Design review of the part built by this model. Coordinates are the model's own, in mm. A direction names the side the tool comes from. Coordinates: 2 decimals unless noted, no trailing zeros. Write each loop counter-clockwise with the first axis right and the second up, starting at its lowest first coordinate (ties: lowest second). Pieces come first, ordered by that corner, then holes. Notation, with made-up numbers: M 89,83 L 132,83 A26 cw 132,119 Z; hole C 77,-22 d10. An arc over 180 degrees is marked long. Write item = value, one per line.
```python
from build123d import *

# Parameters (mm, degrees)
SKETCH_1_W               = 400
SKETCH_1_H               = 150
EXTRUDE_1_DEPTH          = 300
SKETCH_2_R               = 30
EXTRUDE_2_DEPTH          = 20
SKETCH_8_W               = 200
SKETCH_8_H               = 15
EXTRUDE_6_DEPTH          = 80
SKETCH_9_R               = 20
EXTRUDE_7_DEPTH          = 20
MIRROR_4_COPY_1_SKETCH_R = 20
MIRROR_4_COPY_1_DEPTH    = 20
SKETCH_10_R              = 2
CUT_EXTRUDE_1_DEPTH      = 10
EXTRUDE_START            = 20
SKETCH_6_R               = 30
EXTRUDE_8_DEPTH          = 20


with BuildPart() as part:
    # 草图1 → 凸台-拉伸1 (new body)
    with BuildSketch(Plane.XY):
        Rectangle(SKETCH_1_W, SKETCH_1_H)
    extrude(amount=-EXTRUDE_1_DEPTH)

    # 草图2 → 凸台-拉伸2 (add)
    with BuildSketch(Plane(origin=(200, 0, 0), x_dir=(0, 0, -1), z_dir=(1, 0, 0))):
        with Locations(Location((150, 0, 0), (0, 0, 90))):
            Circle(SKETCH_2_R)
    extrude(amount=EXTRUDE_2_DEPTH)

    # 草图8 → 凸台-拉伸6 (add)
    with BuildSketch(Plane.XY):
        with Locations((0, -47.5)):
            Rectangle(SKETCH_8_W, SKETCH_8_H)
    extrude_6 = extrude(amount=EXTRUDE_6_DEPTH)

    # 镜向2: 凸台-拉伸6 across plane
    add(extrude_6.mirror(Plane.XY.offset(-150)))

    # 草图9 → 凸台-拉伸7 (add)
    with BuildSketch(Plane(origin=(100, 0, 0), x_dir=(0, 0, -1), z_dir=(1, 0, 0))):
        with Locations(Location((-80, -47.5, 0), (0, 0, 337.975687163))):
            Circle(SKETCH_9_R)
    extrude_7 = extrude(amount=EXTRUDE_7_DEPTH)

    # 镜向3: 凸台-拉伸7 across plane
    add(extrude_7.mirror(Plane.XY.offset(-150)))

    # 镜向4: 凸台-拉伸7 across plane
    add(extrude_7.mirror(Plane(origin=(0, 0, 0), x_dir=(0, 0, 1), z_dir=(1, 0, 0))))

    # 镜向4 copy 1 sketch → 镜向4 copy 1 (add)
    with BuildSketch(Plane(origin=(-100, 0, -300), x_dir=(0, 0, 1), z_dir=(-1, 0, 0))):
        with Locations(Location((-80, -47.5, 0), (0, 0, 337.975687163))):
            Circle(MIRROR_4_COPY_1_SKETCH_R)
    extrude(amount=MIRROR_4_COPY_1_DEPTH)

    # 草图10 → 切除-拉伸1 (cut)
    with BuildSketch(Plane(origin=(0, 75, 0), x_dir=(1, 0, 0), z_dir=(0, 1, 0))):
        with Locations(Location((0, 187.5, 0), (0, 0, 270))):
            Circle(SKETCH_10_R)
        with Locations(Location((37.5, 150, 0), (0, 0, 270))):
            Circle(SKETCH_10_R)
        with Locations(Location((0, 112.5, 0), (0, 0, 270))):
            Circle(SKETCH_10_R)
        with Locations(Location((-37.5, 150, 0), (0, 0, 270))):
            Circle(SKETCH_10_R)
    extrude(amount=-CUT_EXTRUDE_1_DEPTH, mode=Mode.SUBTRACT)

    # 草图6 → 凸台-拉伸8 (add)
    with BuildSketch(Plane.ZY.offset(200).offset(EXTRUDE_START)):
        with Locations(Location((-150, 0, 0), (0, 0, 90))):
            Circle(SKETCH_6_R)
    extrude(amount=-EXTRUDE_8_DEPTH)


solid = part.part
```
Q1. Consider section C-C, the plane z = -24. State the section outline as (x, y) points, and give its area (3 significant figures).
Check result:
outline = M -200,-75 L 200,-75 L 200,75 L -200,75 Z
area = 60,000 mm²
Q2. The part is to be moulded in two halves that separate along X. For faces 1 (the flat face through (100, -47.1, 80.2)), 2 (the cylindrical face through (209.86, -6.503, -179.287)), 3 (the flat face through (-100, -47.1, 80.2)), 4 (the flat face through (200, -1, -181)), say which applies: +X half, -X half, draft (parallel to the pull), parting line (faces both ways), or undercut.
Check result:
face_1 = undercut
face_2 = draft
face_3 = undercut
face_4 = +X half
Q3. Machinability: for faces 5 (the flat face through (-1, -55, 39)), 6 (the cylindrical face through (-210.14, -6.503, -120.713)), 7 (the flat face through (-120, -47, -380)), 8 (the flat face through (-120, -47, 80)), which of the approach directions +Z, -Z, +X, -X, +Y, -Y give a long, thin tool a straight path to every point of the face, cutting with its end or side? Answer none if there is none.
Check result:
face_5 = +Z, -Y
face_6 = -X
face_7 = -Z, -X, +Y, -Y
face_8 = +Z, -X, +Y, -Y
Q4. Consider section A-A, the plane x = -88. State the section outline as (y, z) points.
Check result:
outline = M -75,-300 L -55,-300 L -55,-380 L -40,-380 L -40,-300 L 75,-300 L 75,0 L -40,0 L -40,80 L -55,80 L -55,0 L -75,0 Z
Q5. Wall thickness on line 1 (X direction, y = 67, z = -150); line 2 (X direction, y = 71, z = -112); line 3 (Z direction, x = -37, y = 69): over which ranges is each line inside the solid? List them lowest first.
Check result:
line_1 = -200 to -39.5, -35.5 to 35.5, 39.5 to 200
line_2 = -200 to -1.94, 1.94 to 200
line_3 = -300 to -151.94, -148.06 to 0
Q6. Consider section D-D, the plane x = -154. State the section outline as (y, z) points.
Check result:
outline = M -75,-300 L 75,-300 L 75,0 L -75,0 Z
Q7. For P1, Ø5, axis at y = -34.5, z = -109, coming from the +X side; P2, Ø10, axis at x = 79, y = -12.5, coming from the +Z side; P3, Ø3, axis at x = 112.5, y = 18.5, coming from the -Z side, all flat-tipped, find the tip position at first contact; note any pin that passes through.
Check result:
P1 = 200
P2 = 0
P3 = -300
Q8. Consider section B-B, the plane y = -47.5. State the section outline as (x, z) points, and give its area (3 significant figures).
Check result:
outline = M -200,-300 L -100,-300 L -100,-360 L -120,-360 L -120,-400 L -100,-400 L -100,-380 L 100,-380 L 100,-400 L 120,-400 L 120,-360 L 100,-360 L 100,-300 L 200,-300 L 200,0 L 100,0 L 100,60 L 120,60 L 120,100 L 100,100 L 100,80 L -100,80 L -100,100 L -120,100 L -120,60 L -100,60 L -100,0 L -200,0 Z
area = 155,000 mm²
